from build123d import *

# Parameters (mm, degrees)
SKETCH_1_W          = 170
SKETCH_1_H          = 72
EXTRUDE_1_DEPTH     = 3
SKETCH_2_W          = 170
SKETCH_2_H          = 72
SKETCH_2_W_2        = 165
SKETCH_2_H_2        = 62
EXTRUDE_2_DEPTH     = 10
SKETCH_3_R          = 1.5
CUT_EXTRUDE_1_DEPTH = 3
SKETCH_4_W          = 29
SKETCH_4_H          = 27
SKETCH_4_W_2        = 8
SKETCH_4_H_2        = 8
CUT_EXTRUDE_2_DEPTH = 3
FILLET_1_R          = 3
SKETCH_5_W          = 11
SKETCH_5_H          = 3
CUT_EXTRUDE_3_DEPTH = 3
FILLET_3_R          = 1
SKETCH_6_W          = 10
SKETCH_6_H          = 5
CUT_EXTRUDE_4_DEPTH = 3
FILLET_4_R          = 1


with BuildPart() as part:
    # 草图1 → 凸台-拉伸1 (new body)
    with BuildSketch(Plane(origin=(0, 0, 0), x_dir=(1, 0, 0), z_dir=(0, 1, 0))):
        Rectangle(SKETCH_1_W, SKETCH_1_H)
    extrude(amount=EXTRUDE_1_DEPTH)

    # 草图2 → 凸台-拉伸2 (add)
    with BuildSketch(Plane(origin=(0, 3, 0), x_dir=(1, 0, 0), z_dir=(0, 1, 0))):
        Rectangle(SKETCH_2_W, SKETCH_2_H)
        Rectangle(SKETCH_2_W_2, SKETCH_2_H_2, mode=Mode.SUBTRACT)
    extrude(amount=EXTRUDE_2_DEPTH)

    # 草图3 → 切除-拉伸1 (cut)
    with BuildSketch(Plane(origin=(0, 13, 0), x_dir=(1, 0, 0), z_dir=(0, 1, 0))):
        with Locations(Location((0, 34, 0), (0, 0, 270))):
            Circle(SKETCH_3_R)
        with Locations(Location((0, -34, 0), (0, 0, 270))):
            Circle(SKETCH_3_R)
    extrude(amount=-CUT_EXTRUDE_1_DEPTH, mode=Mode.SUBTRACT)

    # 草图4 → 切除-拉伸2 (cut)
    with BuildSketch(Plane.XZ):
        with Locations((-6, -9.5)):
            Rectangle(SKETCH_4_W, SKETCH_4_H)
        with Locations((-30.5, -18)):
            Rectangle(SKETCH_4_W_2, SKETCH_4_H_2)
    extrude(amount=-CUT_EXTRUDE_2_DEPTH, mode=Mode.SUBTRACT)

    # 圆角1
    fillet_1_edges = [part.edges().sort_by_distance(p)[0] for p in [
        (0, 0, 36),
        (-85, 0, 0),
        (0, 0, -36),
        (85, 0, 0),
        (85, 6.5, 36),
        (-85, 6.5, 36),
        (-85, 6.5, -36),
        (85, 6.5, -36),
    ]]
    fillet(fillet_1_edges, radius=FILLET_1_R)

    # 草图5 → 切除-拉伸3 (cut)
    with BuildSketch(Plane.ZY.offset(85)):
        with Locations((19.5, 11.5)):
            Rectangle(SKETCH_5_W, SKETCH_5_H)
    extrude(amount=-CUT_EXTRUDE_3_DEPTH, mode=Mode.SUBTRACT)

    # 圆角3
    fillet_3_edges = [part.edges().sort_by_distance(p)[0] for p in [
        (-85, 11.5, 14),
        (-85, 10, 19.5),
        (-85, 11.5, 25),
    ]]
    fillet(fillet_3_edges, radius=FILLET_3_R)

    # 草图6 → 切除-拉伸4 (cut)
    with BuildSketch(Plane(origin=(85, 0, 0), x_dir=(0, 0, -1), z_dir=(1, 0, 0))):
        with Locations((6.5, 7.5)):
            Rectangle(SKETCH_6_W, SKETCH_6_H)
    extrude(amount=-CUT_EXTRUDE_4_DEPTH, mode=Mode.SUBTRACT)

    # 圆角4
    fillet_4_edges = [part.edges().sort_by_distance(p)[0] for p in [
        (85, 7.5, -1.5),
        (85, 5, -6.5),
        (85, 7.5, -11.5),
        (85, 10, -6.5),
    ]]
    fillet(fillet_4_edges, radius=FILLET_4_R)


solid = part.part
Work out the finished part from the listing and answer in its coordinate system (mm). A direction names the side the tool comes from. Give positions to 0.01 mm unless a question says otherwise; leave off trailing zeros. Loops run counter-clockwise (first coordinate to the right, second up) from the corner with the lowest first, then second, coordinate; pieces in that order, holes last. Notation, with made-up numbers: (-30, 58.5) -> (-7, 58.5) arc R10 ccw to (-7, 68.5) -> close; hole circle Ø10 at (78, 32.25). An arc over 180 degrees is marked (long way). Use a Markdown table: item, result. Add a question column.
1. Flat-ended cylindrical pins translate along their axes: pin 1 Ø0.8 at (x, z) = (83.5, -7.5) entering from -Y; pin 2 Ø3 at (x, y) = (21.5, 2) entering from +Z; pin 3 Ø0.9 at (x, z) = (0.5, -34) entering from +Y; pin 4 Ø0.9 at (y, z) = (1, -18.5) entering from +X. Find the tip coordinate at first contact, or state that the pin passes through.
2. Section C-C on y = 7.25 is taken. Determine the outline of the cut face in (x, z).
3. Determine the mould class of faces 1 (the flat face through (85, 8, 0)), 2 (the flat face through (-6, 1, 4)), 3 (the flat face through (0, 13, -32)) for opening direction X: released by +X, released by -X, zero draft, split by the parting line, or undercut.
4. Find the intervals of material crossed by probe 1 along Z at (x, y) = (-28, 6); probe 2 along X at (y, z) = (8.75, 16); probe 3 along Y at (x, z) = (29, 8), in increasing order.
5. Section A-A on x = 0 is taken. Determine the outline of the cut face in (y, z), and give its area (3 significant figures).
6. For faces 4 (the flat face through (-1, 8, -36)), 5 (the flat face through (-1, 8, 31)), 6 (the flat face through (-20.5, 1, -10)), determine the directions among +Z, -Z, +X, -X, +Y, -Y from which every point of the face is accessible in a straight line to the end or side of a thin tool.
7. Section B-B on z = 19 is taken. Determine the outline of the cut face in (x, y), and give its area (3 significant figures).
8. Section D-D on x = -58 is taken. Determine the outline of the cut face in (y, z).
Results below:
| question | item | result |
|---|---|---|
| 1 | pin 1 | stops at y = 0.21 |
| 1 | pin 2 | stops at z = 36 |
| 1 | pin 3 | stops at y = 10 |
| 1 | pin 4 | stops at x = 84.57 |
| 2 | outline | (-85, -33) arc R3 ccw to (-82, -36) -> (82, -36) arc R3 ccw to (85, -33) -> (85, -12.5) arc R1 ccw to (84, -11.5) -> (82.5, -11.5) -> (82.5, -31) -> (-82.5, -31) -> (-82.5, 31) -> (82.5, 31) -> (82.5, -1.5) -> (84, -1.5) arc R1 ccw to (85, -0.5) -> (85, 33) arc R3 ccw to (82, 36) -> (-82, 36) arc R3 ccw to (-85, 33) -> close |
| 3 | face 1 | released by +X |
| 3 | face 2 | undercut |
| 3 | face 3 | zero draft |
| 4 | probe 1 | z = -36 to -31, 31 to 36 |
| 4 | probe 2 | x = -85 to -82.5, 82.5 to 85 |
| 4 | probe 3 | y = 0 to 3 |
| 5 | outline | (0, -33) arc R3 ccw to (3, -36) -> (13, -36) -> (13, -35.5) -> (10, -35.5) -> (10, -32.5) -> (13, -32.5) -> (13, -31) -> (3, -31) -> (3, -23) -> (0, -23) -> close; (0, 4) -> (3, 4) -> (3, 31) -> (13, 31) -> (13, 32.5) -> (10, 32.5) -> (10, 35.5) -> (13, 35.5) -> (13, 36) -> (3, 36) arc R3 ccw to (0, 33) -> close |
| 5 | area | 213 mm^2 |
| 6 | face 4 | -Z, +X, -X, +Y, -Y |
| 6 | face 5 | +Y |
| 6 | face 6 | +Y, -Y |
| 7 | outline | (-85, 3) arc R3 ccw to (-82, 0) -> (82, 0) arc R3 ccw to (85, 3) -> (85, 13) -> (82.5, 13) -> (82.5, 3) -> (-82.5, 3) -> (-82.5, 10) -> (-84, 10) arc R1 ccw to (-85, 9) -> close |
| 7 | area | 548 mm^2 |
| 8 | outline | (0, -33) arc R3 ccw to (3, -36) -> (13, -36) -> (13, -31) -> (3, -31) -> (3, 31) -> (13, 31) -> (13, 36) -> (3, 36) arc R3 ccw to (0, 33) -> close |
